Work out the finished part from the listing and answer in its coordinate system (mm). Round coordinates to 2 decimals unless told otherwise and drop trailing zeros. Loops run counter-clockwise (first coordinate to the right, second up) from the corner with the lowest first, then second, coordinate; pieces in that order, holes last. Notation, with made-up numbers: (1.25, 71) - (24.25, 71) arc R17 cw to (24.25, 79) - close; hole circle Ø2 at (52.25, -10.5). An arc over 180 degrees is marked (long way). Answer as CSV lines item,"result". Start each with the question number.
Q1. Section D-D on x = -0.25 is taken. Write down the section's boundary in (y, z), then the cut area to 3 significant figures.
Q2. Straight lines are drawn through the part: L1, parallel to X at y = -2.45, z = 1; L2, parallel to Z at x = 0, y = -1.15; L3, parallel to X at y = -1.5, z = 1.75. For each, find the intervals that lie inside material, in ascending order. Write a range as [from, to].
Q3. The mould has two halves that part along Z. Classify faces 1 (the face through (-1.16, -2.465, -2.993)), 2 (the face through (9, -2, 3.5)), 3 (the face through (0.27, -2.54, 1.22)): +Z half, -Z half, draft (parallel to the pull), parting line (faces both ways), or undercut.
Q4. Section B-B on y = -1 is taken. Write down the section's boundary in (x, z), then the cut area to 3 significant figures.
Q5. Section C-C on z = 0 is taken. Write down the section's boundary in (x, y), then the cut area to 3 significant figures.
Q6. Section A-A on x = 15 is taken. Write down the section's boundary in (y, z), then the cut area to 3 significant figures.
```python
from build123d import *

# Parameters (mm, degrees)
BLOCK_R                = 2.5
BOSS_EXTRUDE1_DEPTH    = 5
M3_TAPPED_HOLE1_D      = 2.5
M2_TAPPED_HOLE1_REACH  = 21.397
M2_TAPPED_HOLE1_BORE_R = 0.8


with BuildPart() as part:
    # block → Boss-Extrude1 (new body)
    with BuildSketch(Plane(origin=(0, 0, 0), x_dir=(1, 0, 0), z_dir=(0, 1, 0))):
        Polygon((0.732050808, 3.5), (16.5, 3.5), (18.5, 1.5), (18.5, -1.5), (16.5, -3.5), (0.732050808, -3.5), (-3, -2.5), (-3, 2.5), align=None)
        with Locations(Location((15, 0, 0), (0, 0, 270))):
            Circle(BLOCK_R, mode=Mode.SUBTRACT)
    extrude(amount=-BOSS_EXTRUDE1_DEPTH)

    # M3 Tapped Hole1 (through all)
    with Locations(Plane(origin=(0, 0, 0), x_dir=(1, 0, 0), z_dir=(0, 1, 0))):
        with Locations((0, 0)):
            Hole(M3_TAPPED_HOLE1_D / 2)

    # M2 Tapped Hole1 bore → M2 Tapped Hole1 (cut, up to next)
    with BuildSketch(Plane(origin=(10, 0, -10), x_dir=(-0.7071067811865465, 0, -0.7071067811865486), z_dir=(0.7071067811865486, 0, -0.7071067811865465)), mode=Mode.PRIVATE) as m2_tapped_hole1_sk1:
        with Locations((-10.606601718, -2.5)):
            Circle(M2_TAPPED_HOLE1_BORE_R)
    m2_tapped_hole1_tool1 = extrude(m2_tapped_hole1_sk1.sketch, amount=-M2_TAPPED_HOLE1_REACH, mode=Mode.PRIVATE) & part.part
    m2_tapped_hole1 = m2_tapped_hole1_tool1.solids().sort_by_distance((17.5, -2.5, -2.5))[0]
    add(m2_tapped_hole1, mode=Mode.SUBTRACT)

    # Mirror1: M2 Tapped Hole1 across plane
    add(m2_tapped_hole1.mirror(Plane.XY), mode=Mode.SUBTRACT)


solid = part.part
```
Findings:
1,outline,"(-5, -3.24) - (0, -3.24) - (0, -1.22) - (-5, -1.22) - close; (-5, 1.22) - (0, 1.22) - (0, 3.24) - (-5, 3.24) - close"
1,area,"20.1 mm^2"
2,L1,"x = [-3, -0.75], [0.75, 12.71], [17.29, 18.5]"
2,L2,"z = [-3.3, -1.25], [1.25, 3.3]"
2,L3,"x = [-3, 13.21], [16.79, 18.25]"
3,face 1,"-Z half"
3,face 2,"+Z half"
3,face 3,"undercut"
4,outline,"(-3, -2.5) - (0.73, -3.5) - (16.5, -3.5) - (18.5, -1.5) - (18.5, 1.5) - (16.5, 3.5) - (0.73, 3.5) - (-3, 2.5) - close; hole circle Ø2.5 at (0, 0); hole circle Ø5 at (15, 0)"
4,area,"118 mm^2"
5,outline,"(-3, -5) - (-1.25, -5) - (-1.25, 0) - (-3, 0) - close; (1.25, -5) - (12.5, -5) - (12.5, 0) - (1.25, 0) - close; (17.5, -5) - (18.5, -5) - (18.5, 0) - (17.5, 0) - close"
5,area,"70.0 mm^2"
6,outline,"(-5, -3.5) - (0, -3.5) - (0, -2.5) - (-5, -2.5) - close; (-5, 2.5) - (0, 2.5) - (0, 3.5) - (-5, 3.5) - close"
6,area,"10.0 mm^2"
